The listing builds one solid part. Answer for the finished solid, in the listing's coordinates (mm). Face numbers are marked on the shaded views. A direction names the side the tool comes from. Round coordinates to 2 decimals unless told otherwise and drop trailing zeros. Order: outer loops, then holes, each group sorted by start corner. A loop starts at its lowest first (then second) coordinate and runs counter-clockwise, first axis right, second up. Notation, with made-up numbers: M 67,-7.5 L 96,-7.5 A13 cw 96,4.5 Z; hole C 60.25,31.25 d8. An arc over 180 degrees is marked long. Write item = value, one per line. Start each with the question number.
(1) A cutting plane is placed at B-B, the plane y = 0. Determine the outline of the cut face in (x, z), and give its area (3 significant figures).
(2) A cutting plane is placed at C-C, the plane x = 19. Determine the outline of the cut face in (y, z), and give its area (3 significant figures).
(3) Which of the six approach directions +Z, -Z, +X, -X, +Y, -Y give full straight-line access (tool end or side, diameter ignored) to the marked faces 4, 5 and 6?
(4) Straight lines are drawn through the part: probe 1 along Y at (x, z) = (25, 0); probe 2 along X at (y, z) = (3.5, 0); probe 3 along Z at (x, y) = (8.5, 0). For each, find the intervals that lie inside material, in ascending order. Write a range as from..to.
(5) For a pull along Z with two mould halves and no side action, classify the marked faces 1, 2 and 3 as released by +Z, released by -Z, zero draft, split by the parting line, or undercut.
(6) A cutting plane is placed at D-D, the plane x = 9. Determine the outline of the cut face in (y, z).
(7) Each of these flat-tipped pins is pushed along its axis until it touches: pin 1 (6 mm diameter, centred on x = 8.5, z = -1, fed in from +Y); pin 2 (1.9 mm diameter, centred on y = -1, z = 1.5, fed in from -X); pin 3 (8 mm diameter, centred on x = 7.5, z = 6, fed in from -Y). Where does it stop, or does it pass through?
(8) A cutting plane is placed at A-A, the plane z = 0. Determine the outline of the cut face in (x, y).
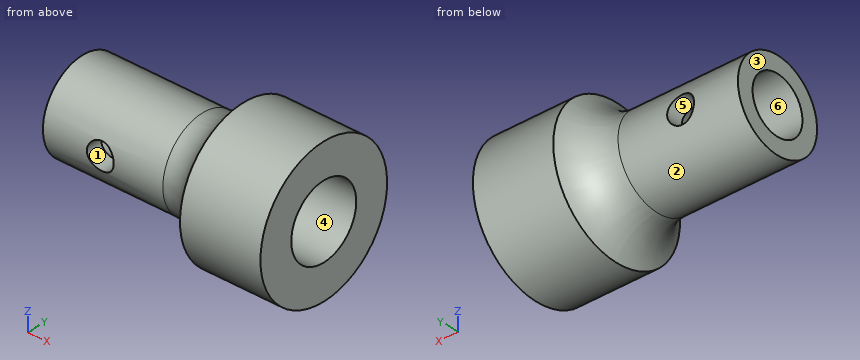
Autodesk Inventor part; units mm, degrees
ref_plane "YZ Plane" through (0, 0, 0) normal (1, 0, 0) x (0, 1, 0)
ref_plane "XZ Plane" through (0, 0, 0) normal (0, 1, 0) x (-1, 0, 0)
ref_plane "XY Plane" through (0, 0, 0) normal (0, 0, 1) x (1, 0, 0)
sketch "Sketch1" plane through (0, 0, 0) normal (1, 0, 0) x (0, 1, 0)
  circle A0 centre (0, 0) radius 3.15
  circle A1 centre (0, 0) radius 5
  dimension "d0" = 6.3
  dimension "d1" = 10
extrude "Extrusion1" add sketch "Sketch1" along normal blind 18
sketch "Sketch2" plane through (18, 0, 0) normal (1, 0, 0) x (0, 0, -1)
  circle A0 centre (0, 0) radius 5
  dimension "d4" = 10
extrude "Extrusion2" add sketch "Sketch2" against normal blind 2
sketch "Sketch3" plane through (18, 0, 0) normal (1, 0, 0) x (0, 0, -1)
  circle A0 centre (0, 0) radius 4.1
  circle A1 centre (0, 0) radius 8
  dimension "d7" = 8.2
  dimension "d8" = 16
extrude "Extrusion3" add sketch "Sketch3" along normal blind 9
fillet "Fillet1" radius 5 1 edges at (18, -5, 0)
sketch "Sketch4" plane through (0, 0, 0) normal (0, 1, 0) x (-1, 0, 0)
  line L0 (-13.4174, 5) -> (-13.4174, -5)
  line L1 (-13.4174, 0) -> (-6.4174, 0)
  circle A0 centre (-6.4174, 0) radius 1.5
  point P0 (0, 0)
  dimension "d12" = 7
  dimension "d13" = 3
extrude "Extrusion4" cut sketch "Sketch4" along normal mid plane 44
properties part number "coupling_motor_lead_screw"
Reported:
q1.outline = M 0,-5 L 13.42,-5 A5 cw 18,-8 L 27,-8 L 27,-4.1 L 18,-4.1 L 18,4.1 L 27,4.1 L 27,8 L 18,8 A5 cw 13.42,5 L 0,5 L 0,3.15 L 16,3.15 L 16,-3.15 L 0,-3.15 Z
q1.area = 157 mm²
q2.outline = C 0,0 d16; hole C 0,0 d8.2
q2.area = 148 mm²
q3.face_4 = +X
q3.face_5 = +Y, -Y
q3.face_6 = -X
q4.probe_1 = -8..-4.1, 4.1..8
q4.probe_2 = 0..4.92, 7.92..18
q4.probe_3 = -5..-3.15, 3.15..5
q5.face_1 = undercut
q5.face_2 = split by the parting line
q5.face_3 = zero draft
q6.outline = C 0,0 d10; hole C 0,0 d6.3
q7.pin_1 = 5
q7.pin_2 = 16
q7.pin_3 = -4.58
q8.outline = M 0,-5 L 4.92,-5 L 4.92,-3.15 L 0,-3.15 Z; M 0,3.15 L 4.92,3.15 L 4.92,5 L 0,5 Z; M 7.92,-5 L 13.42,-5 A5 cw 18,-8 L 27,-8 L 27,-4.1 L 18,-4.1 L 18,4.1 L 27,4.1 L 27,8 L 18,8 A5 cw 13.42,5 L 7.92,5 L 7.92,3.15 L 16,3.15 L 16,-3.15 L 7.92,-3.15 Z
